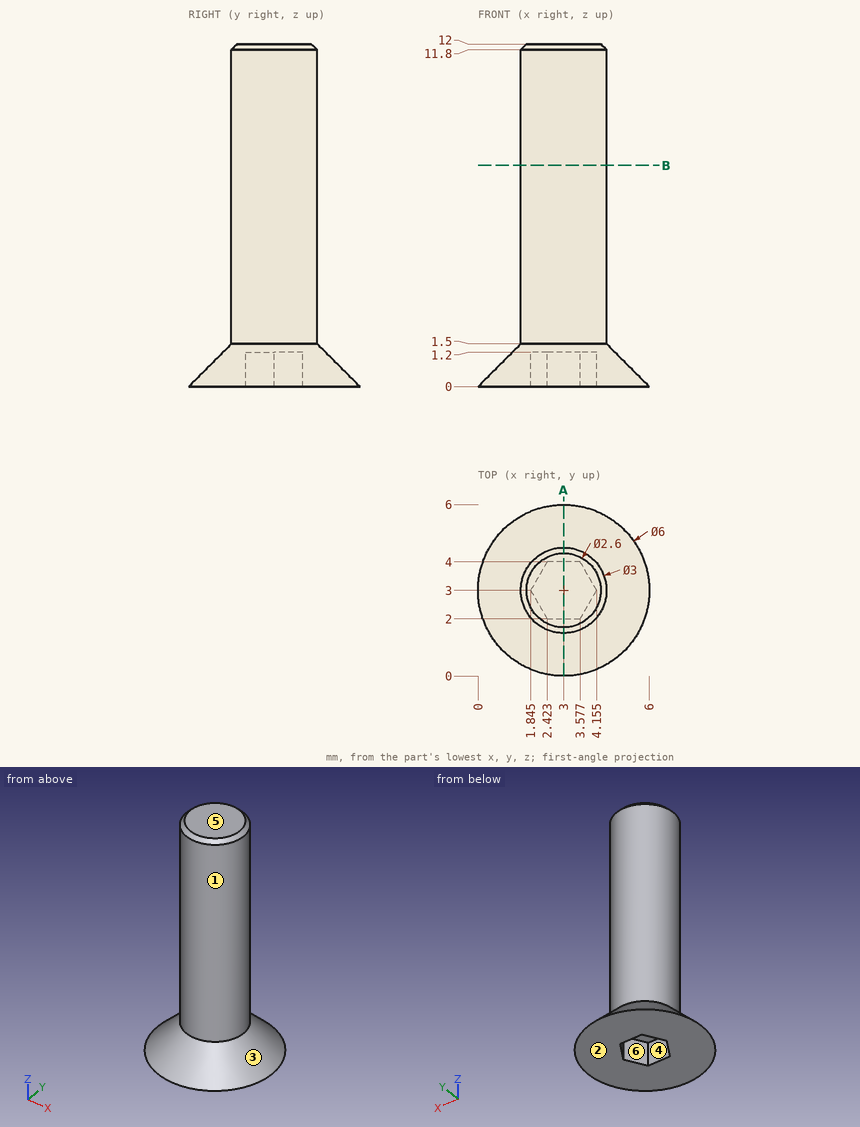
Can you work these out from the drawing? Everything is in mm from the part's minimum corner. A direction names the side the tool comes from. Coordinates: 2 decimals unless noted, no trailing zeros. Loops run counter-clockwise (first coordinate to the right, second up) from the corner with the lowest first, then second, coordinate; pieces in that order, holes last. Notation, with made-up numbers: (-9, 58) - (25, 58) arc R19 cw to (25, 68) - close; hole circle Ø4 at (67, 34.5). An arc over 180 degrees is marked (long way). Use a Markdown table: item, result.
Item 1: We'd pull the mould along Y, two halves only. Please class the marked faces 3, 4, 5 and 6: released by +Y, released by -Y, zero draft, split by the parting line, or undercut.
Numbers:
| item | result |
|---|---|
| face 3 | split by the parting line |
| face 4 | undercut |
| face 5 | zero draft |
| face 6 | undercut |
Item 2: Will these pins go through, and if not, where does the flat tip stop? pin 1 (2 mm diameter, centred on y = 4, z = 2, fed in from +X) (1 decimal); pin 2 (1.5 mm diameter, centred on x = 4, z = 9.5, fed in from +Y); pin 3 (0.6 mm diameter, centred on x = 3, z = 1, fed in from -Y); pin 4 (1 mm diameter, centred on x = 5.5, z = 4.5, fed in from -Y).
Numbers:
| item | result |
|---|---|
| pin 1 | stops at x = 4.8 |
| pin 2 | stops at y = 4.48 |
| pin 3 | stops at y = 0.7 |
| pin 4 | passes through |
Item 3: I want a section at A-A on x = 3. Please give me the cut outline in (y, z).
Numbers:
| item | result |
|---|---|
| outline | (0, 0) - (2, 0) - (2, 1.2) - (4, 1.2) - (4, 0) - (6, 0) - (4.5, 1.5) - (4.5, 11.8) - (4.3, 12) - (1.7, 12) - (1.5, 11.8) - (1.5, 1.5) - close |
Item 4: For the marked faces 1 and 2, which set-ups out of +Z, -Z, +X, -X, +Y, -Y let a thin tool reach every point of the face, with its end or its side?
Numbers:
| item | result |
|---|---|
| face 1 | +Z |
| face 2 | -Z, +X, -X, +Y, -Y |
Item 5: If I drill on probe 1 along Z at (x, y) = (2.9, 2.6); probe 2 along X at (y, z) = (2.9, 5.75); probe 3 along Y at (x, z) = (3.75, 2.75), over which ranges is the centre line in solid material (lowest first)? Write a range as from..to.
Numbers:
| item | result |
|---|---|
| probe 1 | z = 1.2..12 |
| probe 2 | x = 1.5..4.5 |
| probe 3 | y = 1.7..4.3 |
Item 6: I want a section at B-B on z = 7.75. Please give me the cut outline in (x, y).
Numbers:
| item | result |
|---|---|
| outline | circle Ø3 at (3, 3) |
